Could you check a few things on this model? Use its own coordinates, in mm. A direction names the side the tool comes from. Give positions to 0.01 mm unless a question says otherwise; leave off trailing zeros. Write each loop counter-clockwise with the first axis right and the second up, starting at its lowest first coordinate (ties: lowest second). Pieces come first, ordered by that corner, then holes. Notation, with made-up numbers: M 78.25,72 L 126.25,72 A30 cw 126.25,97 Z; hole C 76,-40 d11. An arc over 180 degrees is marked long. Use one line per item in the form item = value.
from build123d import *

# Parameters (mm, degrees)
F1_DEPTH = 25.4
F3_DEPTH = 9.525


with BuildPart() as f1:
    # F0 (on Front) → F1 (new body)
    with BuildSketch(Plane.XZ):
        Polygon((-6.35, 0), (0, 0), (6.35, 0), (3.175, 6.35), (3.175, 9.525), (-3.175, 9.525), (-3.175, 6.35), align=None)
    extrude(amount=F1_DEPTH)

    # F2 (on face) → F3 (join)
    with BuildSketch(Plane.XY.offset(9.525)):
        Polygon((38.1, 0), (0, 0), (-38.1, 0), (-38.1, -12.7), (0, -12.7), (38.1, -12.7), align=None)
    extrude(amount=F3_DEPTH)


solid = f1.part
1) I want a section at C-C, the plane z = 17. Please give me the cut outline in (x, y).
Checked values:
outline = M -38.1,-12.7 L 38.1,-12.7 L 38.1,0 L -38.1,0 Z
2) I want a section at A-A, the plane y = -6. Please give me the cut outline in (x, z) (3 decimals).
Checked values:
outline = M -38.1,9.525 L -3.175,9.525 L -3.175,6.35 L -6.35,0 L 6.35,0 L 3.175,6.35 L 3.175,9.525 L 38.1,9.525 L 38.1,19.05 L -38.1,19.05 Z
3) Thinking about a two-plate mould opening in Z: for faces 1 (the flat face through (-1, -12.7, 14)), 2 (the flat face through (0, -13, 0)), 3 (the flat face through (-4.74, -12.52, 3.22)), 4 (the flat face through (0, -19, 9.525)), which applies, released by +Z, released by -Z, zero draft, split by the parting line, or undercut?
Checked values:
face_1 = zero draft
face_2 = released by -Z
face_3 = undercut
face_4 = released by +Z
4) For faces 5 (the flat face through (4.8, -12.5, 3.1)), 6 (the flat face through (0, -25.4, 4)), 7 (the flat face through (-3.175, -13, 8)), which set-ups out of +Z, -Z, +X, -X, +Y, -Y let a thin tool reach every point of the face, with its end or its side?
Checked values:
face_5 = +X, +Y, -Y
face_6 = +Z, -Z, +X, -X, -Y
face_7 = -X, +Y, -Y
5) I want a section at B-B, the plane x = -27.5. Please give me the cut outline in (y, z) (3 decimals).
Checked values:
outline = M -12.7,9.525 L 0,9.525 L 0,19.05 L -12.7,19.05 Z
6) If I drill on L1, parallel to Z at x = -3, y = -14.5 (3 decimals); L2, parallel to Z at x = 29.5, y = -7.25 (3 decimals); L3, parallel to X at y = -17, z = 9 (3 decimals), over which ranges is the centre line in solid material (lowest first)?
Checked values:
L1 = 0 to 9.525
L2 = 9.525 to 19.05
L3 = -3.175 to 3.175
7) For pin 1 Ø14 at (x, y) = (-20, -3.5) entering from -Z (3 decimals); pin 2 Ø2.5 at (y, z) = (-7.5, 8) entering from -X (3 decimals); pin 3 Ø2 at (x, z) = (14.5, 15.5) entering from -Y, each with a flat end and sliding along its axis, tell me the tip position at first contact or that it passes through.
Checked values:
pin_1 = 9.525
pin_2 = -3.175
pin_3 = -12.7
8) I want a section at D-D, the plane y = -23.5. Please give me the cut outline in (x, z) (3 decimals), plus the area to 3 significant figures.
Checked values:
outline = M -6.35,0 L 6.35,0 L 3.175,6.35 L 3.175,9.525 L -3.175,9.525 L -3.175,6.35 Z
area = 80.6 mm2
